from build123d import *

# Parameters (mm, degrees)
F2_R     = 10
F1_R     = 10
F4_R     = 2
F6_DEPTH = 25


with BuildPart() as f3:
    # F2 (on Front) → F3 section 0
    with BuildSketch(Plane.XZ):
        Circle(F2_R)
    # F1 (on offset) → F3 section 1
    with BuildSketch(Plane.XZ.offset(30)):
        Circle(F1_R)
    loft()

    # F4
    f4_edges = [f3.edges().sort_by_distance(p)[0] for p in [
        (-10, -30, 0),
    ]]
    fillet(f4_edges, radius=F4_R)

    # F5 (on Front) → F6 (cut)
    with BuildSketch(Plane.XZ):
        with BuildLine():
            ThreePointArc((-4.1235491527, 2.8277804697), (-1.4802456276, -4.7758635745), (5, 0))
            ThreePointArc((5, 0), (4.7758635745, 1.4802456276), (4.1235491527, 2.8277804697))
            Line((4.1235491527, 2.8277804697), (-4.1235491527, 2.8277804697))
        make_face()
    extrude(amount=F6_DEPTH, mode=Mode.SUBTRACT)


solid = f3.part
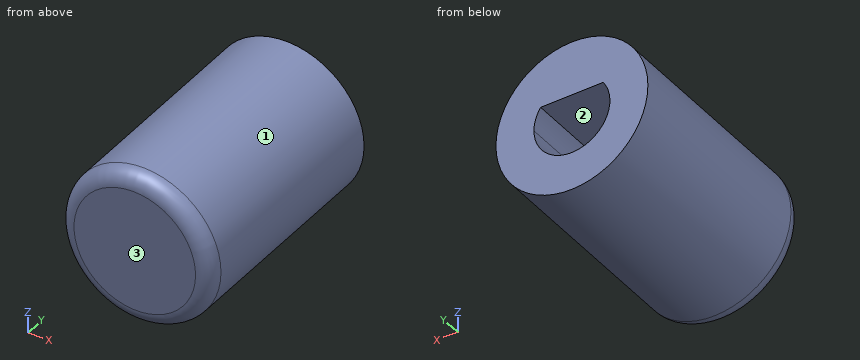
Read the model definition and answer for the solid it produces. Units are mm, in the model's axes. Face numbers are marked on the shaded views. Round coordinates to 2 decimals unless told otherwise and drop trailing zeros. Write each loop counter-clockwise with the first axis right and the second up, starting at its lowest first coordinate (ties: lowest second). Pieces come first, ordered by that corner, then holes.
1. Given pin 1 Ø2 at (y, z) = (-16.5, -1.5) entering from +X; pin 2 Ø1.5 at (x, y) = (-3.5, -16.5) entering from +Z; pin 3 Ø10 at (y, z) = (-16, 7.5) entering from +X, each flat-ended and moving along its own axis, determine where each tip first touches the part or whether it passes through.
2. Determine the mould class of the marked faces 1, 2 and 3 for opening direction X: pulls with the +X half, pulls with the -X half, needs draft (parallel to the pull), parting line crosses it, or undercut.
3. Straight lines are drawn through the part: L1, parallel to Z at x = 0, y = -9; L2, parallel to X at y = -7, z = -0.5; L3, parallel to Y at x = 2, z = -2.25. For each, find the intervals that lie inside material, in ascending order.
4. The part is cut by section A-A, the plane x = 0. Determine the outline of the cut face in (y, z).
5. The part is cut by section B-B, the plane y = -6. Determine the outline of the cut face in (x, z).
Values:
1. pin 1: stops at x = 9.99
1. pin 2: stops at z = 9.61
1. pin 3: stops at x = 9.68
2. face 1: parting line crosses it
2. face 2: undercut
2. face 3: needs draft
3. L1: z = -10 to -5, 2.83 to 10
3. L2: x = -9.99 to -4.97, 4.97 to 9.99
3. L3: y = -30 to -25
4. outline: (-30, -8) arc R2 ccw to (-28, -10) - (0, -10) - (0, -5) - (-25, -5) - (-25, 2.83) - (0, 2.83) - (0, 10) - (-28, 10) arc R2 ccw to (-30, 8) - close
5. outline: circle Ø20 at (0, 0); hole (-4.12, 2.83) arc R5 ccw (long way) to (4.12, 2.83) - close
